Geometry check sheet. Reference: the model listing, model coordinates, mm. A direction names the side the tool comes from. Coordinates: 2 decimals unless noted, no trailing zeros. Loops run counter-clockwise (first coordinate to the right, second up) from the corner with the lowest first, then second, coordinate; pieces in that order, holes last.
from build123d import *

# Parameters (mm, degrees)
SKETCH1_W           = 33.2
SKETCH1_H           = 38
BOSS_EXTRUDE1_DEPTH = 2.75
CUT_EXTRUDE1_DEPTH  = 1.5
SKETCH3_W           = 27.45
SKETCH3_H           = 32
BOSS_EXTRUDE2_DEPTH = 1.5


with BuildPart() as part:
    # Sketch1 → Boss-Extrude1 (new body)
    with BuildSketch(Plane.XY):
        Rectangle(SKETCH1_W, SKETCH1_H)
    extrude(amount=BOSS_EXTRUDE1_DEPTH)

    # Sketch2 → Cut-Extrude1 (cut)
    with BuildSketch(Plane.XY.offset(2.75)):
        Polygon((-6.16774695, -19), (8.23225305, -19), (10.23225305, -17), (13.85, -17), (13.85, -14.655424434), (15.1, -13.405424434), (15.1, 8.4), (13.9, 9.6), (13.9, 11), (16.1, 13.2), (16.1, 18.2), (11.4, 18.2), (11.4, 19), (-10.6, 19), (-10.6, 15.4), (-14, 15.4), (-14, 12.4), (-15.1, 11.3), (-15.1, -13.45), (-13.85, -14.7), (-13.85, -17), (-8.16774695, -17), align=None)
    extrude(amount=-CUT_EXTRUDE1_DEPTH, mode=Mode.SUBTRACT)

    # Sketch3 → Boss-Extrude2 (add)
    with BuildSketch(Plane.XY.offset(1.25)):
        with Locations((-0.075, -0.8)):
            Rectangle(SKETCH3_W, SKETCH3_H)
    extrude(amount=BOSS_EXTRUDE2_DEPTH)


solid = part.part
(1) Sectioned sample at B-B on x = -5. Record the cut outline in (y, z).
Findings:
outline: (-19, 0) - (19, 0) - (19, 1.25) - (15.2, 1.25) - (15.2, 2.75) - (-16.8, 2.75) - (-16.8, 1.25) - (-19, 1.25) - close
(2) Scan lines: L1, parallel to X at y = 15, z = 1.6; L2, parallel to X at y = 15.5, z = 2.65; L3, parallel to X at y = -12.5, z = 1.95. Record each from-to range of solid material in increasing order.
Findings:
L1: x = -16.6 to -14, -13.8 to 13.65, 16.1 to 16.6
L2: x = -16.6 to -10.6, 16.1 to 16.6
L3: x = -16.6 to -15.1, -13.8 to 13.65, 15.1 to 16.6
(3) Draft check along Y on faces 1 (the flat face through (-14.48, -14.07, 2.01)), 2 (the flat face through (14, 18.2, 2)), 3 (the flat face through (0, -1, 2.75)). Enter one of: +Y half, -Y half, draft (parallel to the pull), parting line (faces both ways), or undercut.
Findings:
face 1: undercut
face 2: undercut
face 3: draft
(4) Access from +Z, -Z, +X, -X, +Y, -Y to the whole of each face (thin tool, end or side, straight path). Record for faces 4 (the flat face through (0, 0, 0)), 5 (the flat face through (14.5, 9, 2)).
Findings:
face 4: -Z, +X, -X, +Y, -Y
face 5: +Z
(5) Gauge pin test, flat ends, axial feed: pin 1 Ø0.8 at (x, z) = (-0.5, 2) entering from -Y; pin 2 Ø0.8 at (x, z) = (-2, 2) entering from +Y. Record the tip position at first contact, or that the pin passes through.
Findings:
pin 1: stops at y = -16.8
pin 2: stops at y = 15.2
(6) Sectioned sample at A-A on y = -1. Record the cut outline in (x, z), and give its area (3 significant figures).
Findings:
outline: (-16.6, 0) - (16.6, 0) - (16.6, 2.75) - (15.1, 2.75) - (15.1, 1.25) - (13.65, 1.25) - (13.65, 2.75) - (-13.8, 2.75) - (-13.8, 1.25) - (-15.1, 1.25) - (-15.1, 2.75) - (-16.6, 2.75) - close
area: 87.2 mm2
